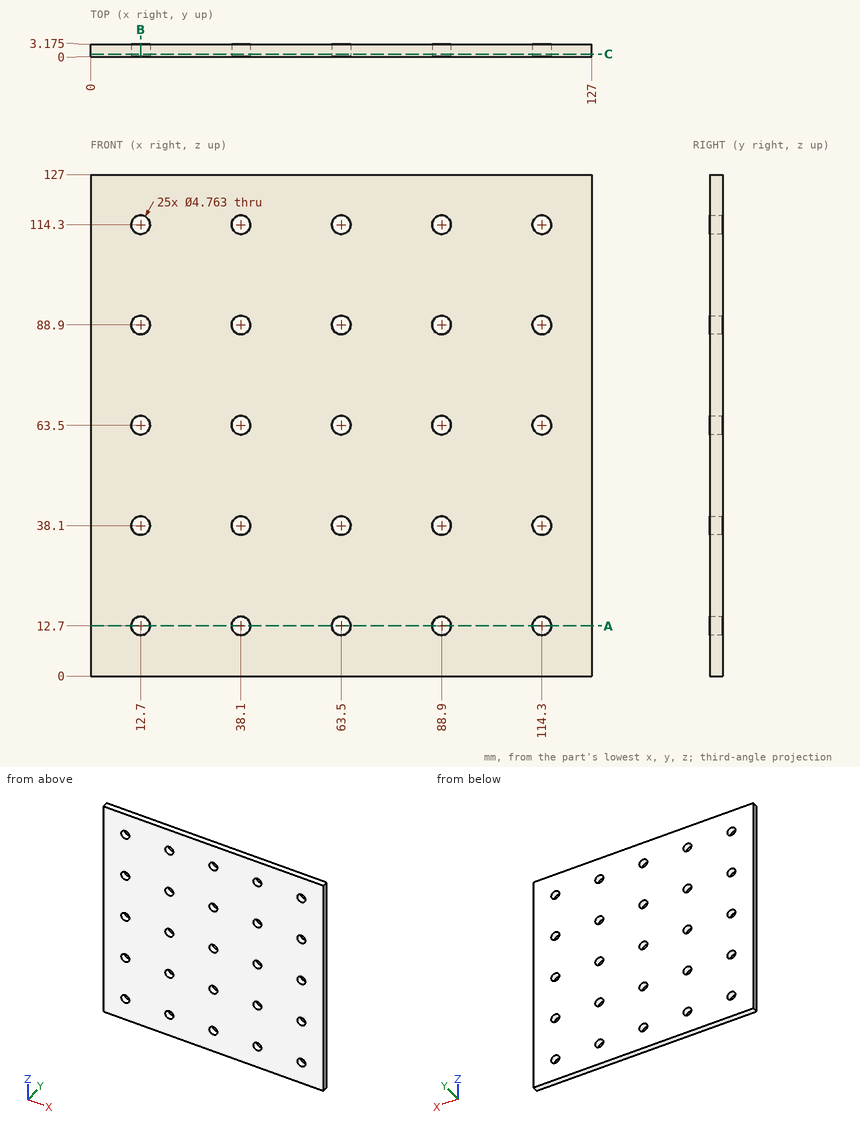
Input: dimensioned drawing with shaded views. Units: mm. Origin: part minimum x, y, z. Coordinates: 2 decimals unless noted, no trailing zeros. Order: outer loops, then holes, each group sorted by start corner. A loop starts at its lowest first (then second) coordinate and runs counter-clockwise, first axis right, second up. Notation, with made-up numbers: (54, 17.25) -> (94, 17.25) arc R14 cw to (94, 30.25) -> close; hole circle Ø4 at (1, 58.5). An arc over 180 degrees is marked (long way). Answer in a Markdown table with one row per item.
Item 1: Contact query for a flat-ended pin moving along its axis: P1, Ø3, axis at x = 88.9, z = 63.5, coming from the -Y side. Output: stop coordinate, or through.
Return value:
| item | result |
|---|---|
| P1 | passes through |
Item 2: Section B-B on x = 12.7. Output: boundary loops of the cut face in (y, z) (1 decimal).
Return value:
| item | result |
|---|---|
| outline | (0, 0) -> (3.2, 0) -> (3.2, 10.3) -> (0, 10.3) -> close; (0, 15.1) -> (3.2, 15.1) -> (3.2, 35.7) -> (0, 35.7) -> close; (0, 40.5) -> (3.2, 40.5) -> (3.2, 61.1) -> (0, 61.1) -> close; (0, 65.9) -> (3.2, 65.9) -> (3.2, 86.5) -> (0, 86.5) -> close; (0, 91.3) -> (3.2, 91.3) -> (3.2, 111.9) -> (0, 111.9) -> close; (0, 116.7) -> (3.2, 116.7) -> (3.2, 127) -> (0, 127) -> close |
Item 3: Ray query, L1, parallel to X at y = 2.4, z = 88.9. Return the intervals inside material, ascending.
Return value:
| item | result |
|---|---|
| L1 | x = 0 to 10.32, 15.08 to 35.72, 40.48 to 61.12, 65.88 to 86.52, 91.28 to 111.92, 116.68 to 127 |
Item 4: Section A-A on z = 12.7. Output: boundary loops of the cut face in (x, y) (1 decimal).
Return value:
| item | result |
|---|---|
| outline | (0, 0) -> (10.3, 0) -> (10.3, 3.2) -> (0, 3.2) -> close; (15.1, 0) -> (35.7, 0) -> (35.7, 3.2) -> (15.1, 3.2) -> close; (40.5, 0) -> (61.1, 0) -> (61.1, 3.2) -> (40.5, 3.2) -> close; (65.9, 0) -> (86.5, 0) -> (86.5, 3.2) -> (65.9, 3.2) -> close; (91.3, 0) -> (111.9, 0) -> (111.9, 3.2) -> (91.3, 3.2) -> close; (116.7, 0) -> (127, 0) -> (127, 3.2) -> (116.7, 3.2) -> close |
Item 5: Section C-C on y = 0.6. State how many separate pieces and enclosed holes the cut face has, plus the area to 3 significant figures.
Return value:
| item | result |
|---|---|
| separate pieces | 1 |
| enclosed holes | 25 |
| area | 15,700 mm² |
